CAD build for the part. Positions are in the model's coordinates, mm. Give positions to 0.01 mm unless a question says otherwise; leave off trailing zeros. Write each loop counter-clockwise with the first axis right and the second up, starting at its lowest first coordinate (ties: lowest second). Pieces come first, ordered by that corner, then holes. Notation, with made-up numbers: (72, -8.5) -> (88, -8.5) arc R36 cw to (88, 30.5) -> close; hole circle Ø11 at (-15.75, -32). An arc over 180 degrees is marked (long way). Answer as a JSON object with one key per item and string values.
```python
from build123d import *

# Parameters (mm, degrees)
SKETCH_1_W      = 235
SKETCH_1_H      = 90
EXTRUDE_1_DEPTH = 3
EXTRUDE_2_DEPTH = 20


with BuildPart() as part:
    # 草图1 → 凸台-拉伸1 (new body)
    with BuildSketch(Plane.XY):
        Rectangle(SKETCH_1_W, SKETCH_1_H)
    extrude(amount=EXTRUDE_1_DEPTH)

    # 草图2 → 凸台-拉伸2 (add)
    with BuildSketch(Plane.ZY.offset(117.5)):
        with BuildLine():
            Line((0.75, 2.25), (2.25, 2.25))
            Line((2.25, 2.25), (2.25, 1.299038106))
            ThreePointArc((2.25, 1.299038106), (1.5, -1.5), (0.75, 1.299038106))
            Line((0.75, 1.299038106), (0.75, 2.25))
        make_face()
    extrude(amount=EXTRUDE_2_DEPTH)


solid = part.part
```
1) Slice it at A-A (z = 1.5). List the corners of the cut face in (x, y), then the cut area to 3 significant figures.
Model answer:
{"outline": "(-137.5, -1.5) -> (-117.5, -1.5) -> (-117.5, -45) -> (117.5, -45) -> (117.5, 45) -> (-117.5, 45) -> (-117.5, 2.25) -> (-137.5, 2.25) -> close", "area": "21,200 mm2"}
2) Pin check, flat tips, straight feed: pin 1 (0.5 mm diameter, centred on x = -127.5, y = 2, fed in from +Z); pin 2 (1.5 mm diameter, centred on y = 19, z = 1, fed in from -X); pin 3 (1.6 mm diameter, centred on x = -127, z = 2, fed in from +Y). Stop position of each tip, or through.
Model answer:
{"pin 1": "stops at z = 2.25", "pin 2": "stops at x = -117.5", "pin 3": "stops at y = 2.25"}
3) Slice it at B-B (y = -21.5). List the corners of the cut face in (x, z).
Model answer:
{"outline": "(-117.5, 0) -> (117.5, 0) -> (117.5, 3) -> (-117.5, 3) -> close"}
4) Wall check: probe 1 along X at (y, z) = (-6.5, 1.8). Give the ranges that are in metal, low to high.
Model answer:
{"probe 1": "x = -117.5 to 117.5"}
